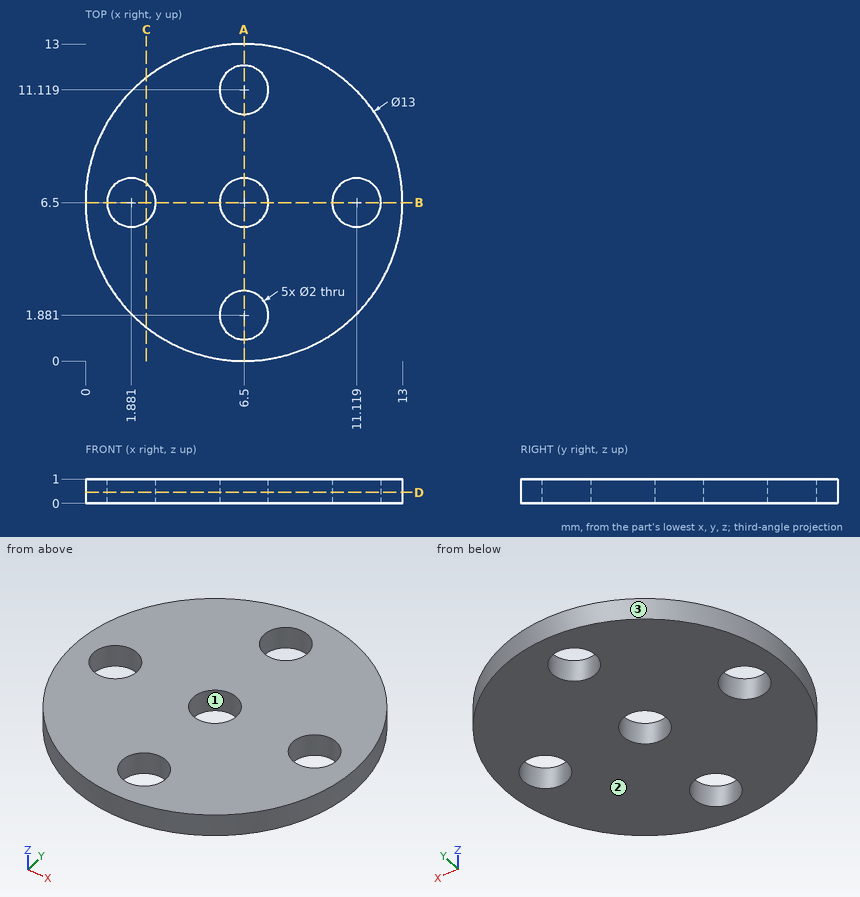
Input: dimensioned drawing with shaded views. Units: mm. Origin: part minimum x, y, z. Coordinates: 2 decimals unless noted, no trailing zeros. Loops run counter-clockwise (first coordinate to the right, second up) from the corner with the lowest first, then second, coordinate; pieces in that order, holes last. Notation, with made-up numbers: M 44.25,35.25 L 100.25,35.25 A34 ccw 100.25,72.25 Z; hole C -21,18.5 d4. An arc over 180 degrees is marked long. One line per item, written item: value. Start each with the question number.
1) Material intervals for L1, parallel to Y at x = 6.5, z = 0.35; L2, parallel to Y at x = 7.25, z = 0.3 (1 decimal); L3, parallel to Y at x = 11.75, z = 0.3 (1 decimal), sorted ascending. Write a range as from..to.
2) Cut plane D-D (z = 0.45). Return loops of the section in (x, y).
3) Cut plane C-C (x = 2.5). Return loops of the section in (y, z) (1 decimal).
4) Pin query (flat end, axial travel): P1, Ø1.8, axis at x = 1.88, y = 6.5, coming from the +Z side. Return the tip coordinate at first contact, or that it passes through.
5) Cut plane A-A (x = 6.5). Return loops of the section in (y, z).
6) Draft query along Y for the marked faces 1, 2 and 3. Return one class per face: released by +Y, released by -Y, zero draft, split by the parting line, or undercut.
Evaluation:
1. L1: 0..0.88, 2.88..5.5, 7.5..10.12, 12.12..13
1. L2: 0..1.2, 2.5..5.8, 7.2..10.5, 11.8..13
1. L3: 2.7..5.7, 7.3..10.3
2. outline: C 6.5,6.5 d13; hole C 1.88,6.5 d2; hole C 6.5,1.88 d2; hole C 6.5,6.5 d2; hole C 6.5,11.12 d2; hole C 11.12,6.5 d2
3. outline: M 1.4,0 L 5.7,0 L 5.7,1 L 1.4,1 Z; M 7.3,0 L 11.6,0 L 11.6,1 L 7.3,1 Z
4. P1: through
5. outline: M 0,0 L 0.88,0 L 0.88,1 L 0,1 Z; M 2.88,0 L 5.5,0 L 5.5,1 L 2.88,1 Z; M 7.5,0 L 10.12,0 L 10.12,1 L 7.5,1 Z; M 12.12,0 L 13,0 L 13,1 L 12.12,1 Z
6. face 1: undercut
6. face 2: zero draft
6. face 3: split by the parting line
